Model file for the job. Use its own axes, mm. Face numbers are marked on the shaded views. A direction names the side the tool comes from. Coordinates: 2 decimals unless noted, no trailing zeros. Write each loop counter-clockwise with the first axis right and the second up, starting at its lowest first coordinate (ties: lowest second). Pieces come first, ordered by that corner, then holes.
Q1. Band-saw the part on A-A, the plane y = 0. Write the cut outline in (x, z).
Q2. Drill centre lines: probe 1 along Y at (x, z) = (-7.75, 19.65); probe 2 along Z at (x, y) = (-8.5, -9.5); probe 3 along Z at (x, y) = (0.5, 16.5). Where is each one in solid material? Low to high.
Q3. Band-saw the part on D-D, the plane x = -15.5. Write the cut outline in (y, z).
Q4. Pin check, flat tips, straight feed: P1, Ø1.5, axis at x = -15.5, y = 0.5, coming from the +Z side; P2, Ø1, axis at y = 3.5, z = 15, coming from the +X side; P3, Ø4, axis at y = 10, z = 13.5, coming from the +X side. Stop position of each tip, or through.
Q5. Band-saw the part on B-B, the plane x = 12. Write the cut outline in (y, z), plus the area to 3 significant figures.
Q6. Which spindle directions (+Z, -Z, +X, -X, +Y, -Y) get a long thin tool onto all of the face, cutting with end or side? Do the marked faces 1, 2 and 3. Say none if no direction does.
Q7. Band-saw the part on C-C, the plane z = 33.5. Write the cut outline in (x, y), plus the area to 3 significant figures.
from build123d import *

# Parameters (mm, degrees)
SKETCH1_R               = 18.4
BOSS_EXTRUDE1_DEPTH     = 22
SKETCH2_R               = 17.4
BOSS_EXTRUDE2_DEPTH     = 30
SKETCH3_R               = 6
BOSS_EXTRUDE3_DEPTH     = 6.5
CHAMFER1_SIZE           = 1
SKETCH4_R               = 3
BOSS_EXTRUDE4_DEPTH     = 15.5
SKETCH5_W               = 12
SKETCH5_H               = 0.6
CUT_EXTRUDE1_DEPTH      = 15.5
CUT_EXTRUDE1_DEPTH_BACK = 15.5
SKETCH6_R               = 1.5
CUT_EXTRUDE2_DEPTH      = 5
SKETCH7_R               = 9.168264785
BOSS_EXTRUDE5_DEPTH     = 12.5
SKETCH8_R               = 14.168264785
BOSS_EXTRUDE6_DEPTH     = 5


with BuildPart() as part:
    # Sketch1 → Boss-Extrude1 (new body)
    with BuildSketch(Plane.XY):
        Circle(SKETCH1_R)
    extrude(amount=BOSS_EXTRUDE1_DEPTH)

    # Sketch2 → Boss-Extrude2 (add)
    with BuildSketch(Plane(origin=(0, 0, 0), x_dir=(-1, 0, 0), z_dir=(0, 0, -1))):
        Circle(SKETCH2_R)
    extrude(amount=BOSS_EXTRUDE2_DEPTH)

    # Sketch3 → Boss-Extrude3 (add)
    with BuildSketch(Plane.XY.offset(22)):
        with Locations((0, -7)):
            Circle(SKETCH3_R)
    extrude(amount=BOSS_EXTRUDE3_DEPTH)

    # Chamfer1
    chamfer1_edges = [part.edges().sort_by_distance(p)[0] for p in [
        (-6, -7, 28.5),
    ]]
    chamfer(chamfer1_edges, length=CHAMFER1_SIZE)

    # Sketch4 → Boss-Extrude4 (add)
    with BuildSketch(Plane.XY.offset(28.5)):
        with Locations((0, -7)):
            Circle(SKETCH4_R)
    extrude(amount=BOSS_EXTRUDE4_DEPTH)

    # Sketch5 → Cut-Extrude1 (cut, two sides)
    with BuildSketch(Plane(origin=(0, 0, 0), x_dir=(0, 0, -1), z_dir=(1, 0, 0))) as cut_extrude1_sk:
        with Locations((-38, -4.3)):
            Rectangle(SKETCH5_W, SKETCH5_H)
    extrude(amount=CUT_EXTRUDE1_DEPTH, mode=Mode.SUBTRACT)
    extrude(cut_extrude1_sk.sketch, amount=-CUT_EXTRUDE1_DEPTH_BACK, mode=Mode.SUBTRACT)

    # Sketch6 → Cut-Extrude2 (cut)
    with BuildSketch(Plane.XY.offset(22)):
        with Locations((-7.75, 13.423393759)):
            Circle(SKETCH6_R)
        with Locations((7.75, 13.423393759)):
            Circle(SKETCH6_R)
        with Locations((15.5, 0)):
            Circle(SKETCH6_R)
        with Locations((-15.5, 0)):
            Circle(SKETCH6_R)
        with Locations((-7.75, -13.423393759)):
            Circle(SKETCH6_R)
        with Locations((7.75, -13.423393759)):
            Circle(SKETCH6_R)
    extrude(amount=-CUT_EXTRUDE2_DEPTH, mode=Mode.SUBTRACT)

    # Sketch7 → Boss-Extrude5 (add)
    with BuildSketch(Plane(origin=(0, 0, -30), x_dir=(-1, 0, 0), z_dir=(0, 0, -1))):
        Circle(SKETCH7_R)
    extrude(amount=BOSS_EXTRUDE5_DEPTH)

    # Sketch8 → Boss-Extrude6 (add)
    with BuildSketch(Plane(origin=(0, 0, -30), x_dir=(-1, 0, 0), z_dir=(0, 0, -1))):
        Circle(SKETCH8_R)
    extrude(amount=BOSS_EXTRUDE6_DEPTH)


solid = part.part
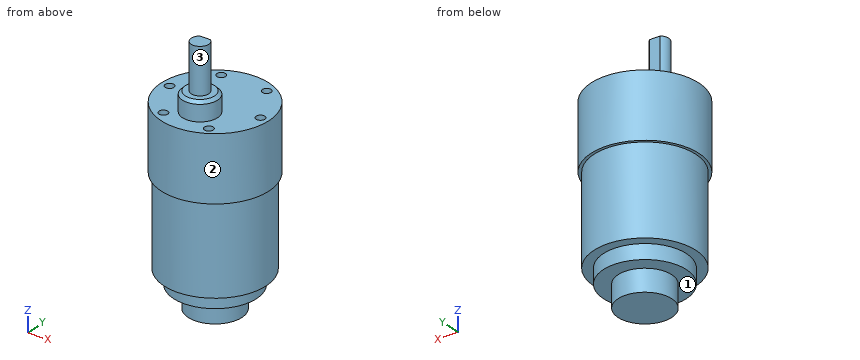
Answer sheet:
1. outline: (-18.4, 0) - (-17.4, 0) - (-17.4, -30) - (-14.17, -30) - (-14.17, -35) - (-9.17, -35) - (-9.17, -42.5) - (9.17, -42.5) - (9.17, -35) - (14.17, -35) - (14.17, -30) - (17.4, -30) - (17.4, 0) - (18.4, 0) - (18.4, 22) - (17, 22) - (17, 17) - (14, 17) - (14, 22) - (-14, 22) - (-14, 17) - (-17, 17) - (-17, 22) - (-18.4, 22) - close
2. probe 1: y = -16.69 to -14.92, -11.92 to 11.92, 14.92 to 16.69
2. probe 2: z = -35 to 22
2. probe 3: z = -30 to 22
3. outline: (-9.92, 0) - (-7.91, 0) - (-7.91, -30) - (7.91, -30) - (7.91, 0) - (9.92, 0) - (9.92, 22) - (1.5, 22) - (1.5, 17) - (-1.5, 17) - (-1.5, 22) - (-9.92, 22) - close
4. P1: stops at z = 17
4. P2: stops at x = 18.15
4. P3: stops at x = 16.57
5. outline: (-13.95, 0) - (-12.6, 0) - (-12.6, -30) - (-7.53, -30) - (-7.53, -35) - (7.53, -35) - (7.53, -30) - (12.6, -30) - (12.6, 0) - (13.95, 0) - (13.95, 22) - (-13.95, 22) - close
5. area: 1,450 mm2
6. face 1: -Z
6. face 2: +Z, -Z
6. face 3: +Z
7. outline: (-1.8, -4.6) arc R3 ccw (long way) to (1.8, -4.6) - close
7. area: 26.8 mm2
